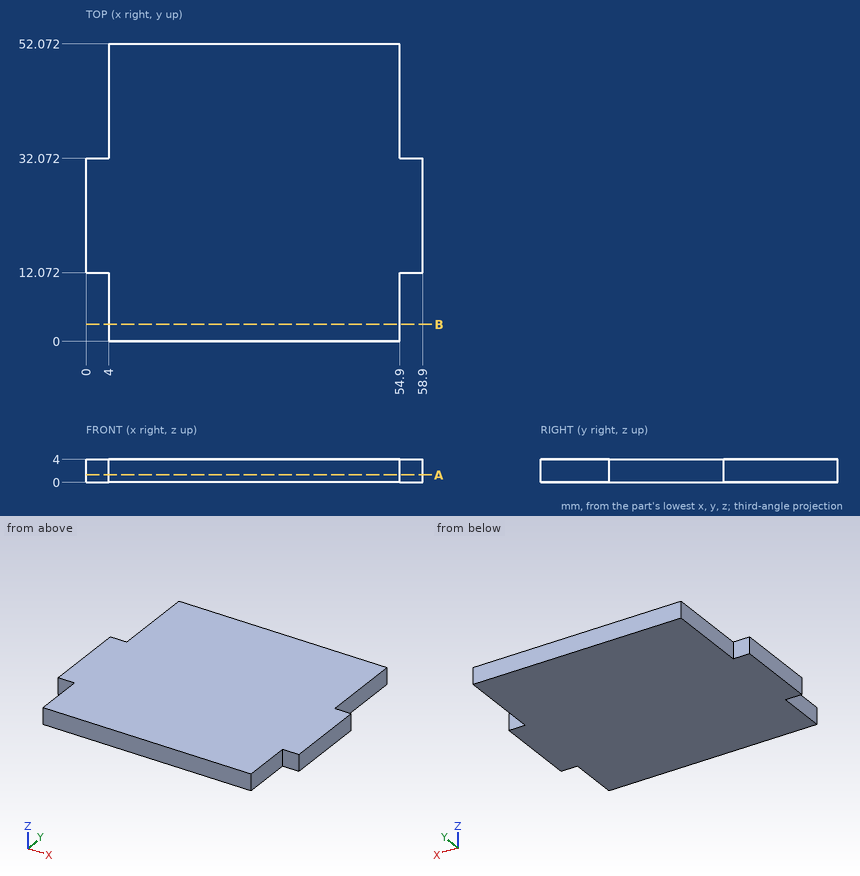
Answer from the drawing. Dimensions are ordinates in mm from the lowest x, y and z of the part. Coordinates: 2 decimals unless noted, no trailing zeros. Order: outer loops, then holes, each group sorted by start corner. A loop starts at its lowest first (then second) coordinate and runs counter-clockwise, first axis right, second up. Notation, with made-up numbers: (68, -4) - (105, -4) arc R31 cw to (105, 35) - close; hole circle Ø5 at (-23.5, -39). An arc over 180 degrees is marked (long way). Put each result on its own line as item: value. Start each with the question number.
1) Find section A-A (z = 1.3). Give the vertices of the cut face in (x, y).
2) Flat-ended cylindrical pins translate along their axes: pin 1 (1 mm diameter, centred on y = 8, z = 2, fed in from -X); pin 2 (1.2 mm diameter, centred on y = 40.5, z = 2.5, fed in from +X); pin 3 (1 mm diameter, centred on x = 50, z = 0.5, fed in from -Y). Find the tip coordinate at first contact, or state that the pin passes through.
3) Find the intervals of material crossed by line 1 (X direction, y = 49.5, z = 1.15), in increasing order. Write a range as from..to.
4) Find section B-B (y = 3). Give the vertices of the cut face in (x, z).
Results list:
1. outline: (0, 12.07) - (4, 12.07) - (4, 0) - (54.9, 0) - (54.9, 12.07) - (58.9, 12.07) - (58.9, 32.07) - (54.9, 32.07) - (54.9, 52.07) - (4, 52.07) - (4, 32.07) - (0, 32.07) - close
2. pin 1: stops at x = 4
2. pin 2: stops at x = 54.9
2. pin 3: stops at y = 0
3. line 1: x = 4..54.9
4. outline: (4, 0) - (54.9, 0) - (54.9, 4) - (4, 4) - close
